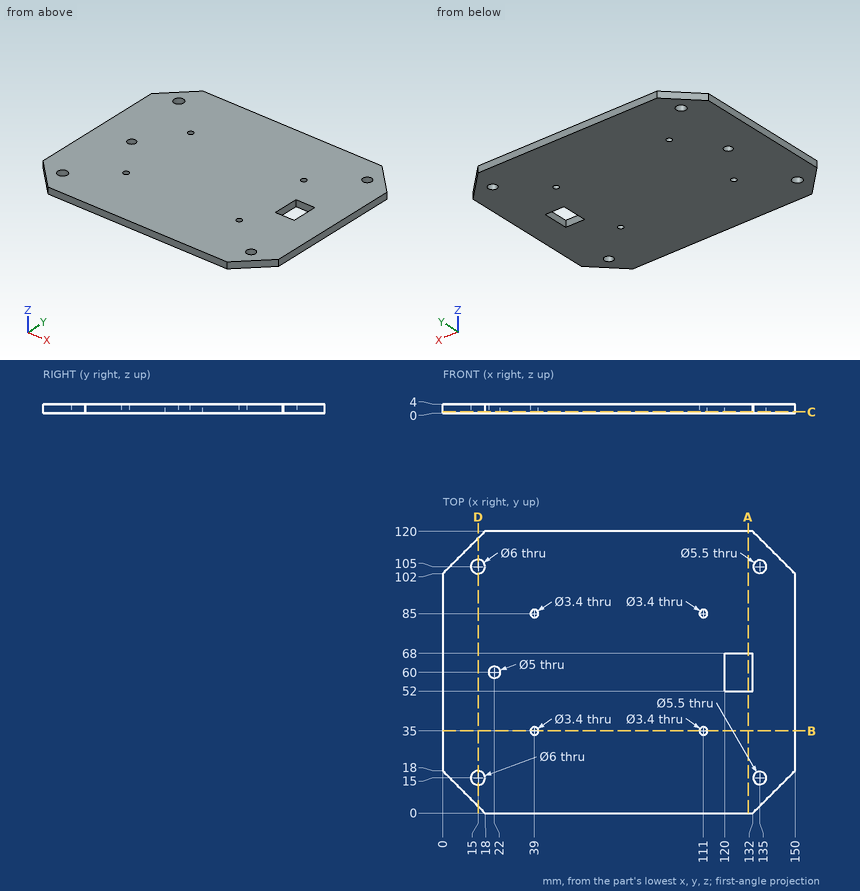
The figure shows three views and two pictorial views of one solid part (mm, origin at its lowest corner). Answer the questions. Round coordinates to 2 decimals unless told otherwise and drop trailing zeros. Write each loop counter-clockwise with the first axis right and the second up, starting at its lowest first coordinate (ties: lowest second). Pieces come first, ordered by that corner, then holes. Notation, with made-up numbers: (-7, 89.25) - (48, 89.25) arc R12 cw to (48, 96.25) - close; hole circle Ø10 at (79, -38.5). An arc over 180 degrees is marked (long way). One line per question, with ' | ' between items. Start each with the question number.
1. Find the intervals of material crossed by probe 1 along Y at (x, z) = (135, 2.75); probe 2 along X at (y, z) = (56, 2.45); probe 3 along Y at (x, z) = (22, 2.3), in increasing order. Write a range as [from, to].
2. Section C-C (z = 0.6) is taken. Give the number of separate pieces and of enclosed holes in the cut face, and give its area (3 significant figures).
3. Section D-D (x = 15) is taken. Determine the outline of the cut face in (y, z), and give its area (3 significant figures).
4. Section A-A (x = 130) is taken. Determine the outline of the cut face in (y, z).
5. Section B-B (y = 35) is taken. Determine the outline of the cut face in (x, z), and give its area (3 significant figures).
Filled in:
1) probe 1: [3, 12.25], [17.75, 102.25], [107.75, 117] | probe 2: [0, 120], [132, 150] | probe 3: [0, 57.5], [62.5, 120]
2) separate pieces: 1 | enclosed holes: 10 | area: 17,000 mm²
3) outline: (3, 0) - (12, 0) - (12, 4) - (3, 4) - close; (18, 0) - (102, 0) - (102, 4) - (18, 4) - close; (108, 0) - (117, 0) - (117, 4) - (108, 4) - close | area: 408 mm²
4) outline: (0, 0) - (52, 0) - (52, 4) - (0, 4) - close; (68, 0) - (120, 0) - (120, 4) - (68, 4) - close
5) outline: (0, 0) - (37.3, 0) - (37.3, 4) - (0, 4) - close; (40.7, 0) - (109.3, 0) - (109.3, 4) - (40.7, 4) - close; (112.7, 0) - (150, 0) - (150, 4) - (112.7, 4) - close | area: 573 mm²
